Could you check a few things on this model? Use its own coordinates, in mm. A direction names the side the tool comes from. Coordinates: 2 decimals unless noted, no trailing zeros. Write each loop counter-clockwise with the first axis right and the second up, starting at its lowest first coordinate (ties: lowest second). Pieces come first, ordered by that corner, then holes.
Item 1: Thinking about a two-plate mould opening in Y: for faces 4 (the flat face through (-38.1, 65.4, 39.9)), 5 (the cylindrical face through (-31.839, -60.47, -46.367)), which applies, +Y half, -Y half, draft (parallel to the pull), parting line (faces both ways), or undercut?
Item 2: For P1, Ø12, axis at y = 63.5, z = -82.5, coming from the +X side; P2, Ø1.5, axis at x = -15.5, y = 2, coming from the -Z side; P3, Ø2, axis at x = 11.5, y = -23, coming from the -Z side; P4, Ø9.5, axis at y = 0, z = 0, coming from the -X side, each with a flat end and sliding along its axis, tell me the tip position at first contact or that it passes through.
Item 3: If I drill on probe 1 along X at (y, z) = (-67, 24.5); probe 2 along Z at (x, y) = (31.5, 0); probe 3 along X at (y, z) = (60, -67), over which ranges is the centre line in solid material (lowest first)?
Item 4: I want a section at C-C on x = -13.5. Please give me the cut outline in (y, z) (1 decimal), then the cut area to 3 significant figures.
Item 5: Which directions (+Z, -Z, +X, -X, +Y, -Y) give clear straight access to the entire face, cutting with the end or side of a thin tool? Please do faces 1 (the cylindrical face through (31.661, -60.47, -46.367)), 2 (the flat face through (-25.4, 16, 1)), 3 (the flat face through (38.1, 65.4, 39.9)).
from build123d import *

# Parameters (mm, degrees)
F0_R     = 127
F0_R_2   = 76.2
F1_DEPTH = 38.1
F2_R     = 38.09999
F0_R_3   = 7.9375
F3_DEPTH = 25.4


# Not quite as in the source:
# - a fillet or chamfer is up to 0.001 mm smaller than in the source, because OpenCascade refuses the exact size


with BuildPart() as f1:
    # F0 (on Right) → F1 (new body, symmetric)
    with BuildSketch(Plane.YZ):
        Circle(F0_R)
        Circle(F0_R_2, mode=Mode.SUBTRACT)
    extrude(amount=F1_DEPTH, both=True)

    # F2 (radius 38.1 in the source; OpenCascade refuses exactly that, so slightly less here)
    f2_edges = [f1.edges().sort_by_distance(p)[0] for p in [
        (38.1, -127, 0),
        (-38.1, -127, 0),
    ]]
    fillet(f2_edges, radius=F2_R)

    # F0 (on Right) → F3 (join, symmetric)
    with BuildSketch(Plane.YZ):
        Circle(F0_R_2)
        Circle(F0_R_3, mode=Mode.SUBTRACT)
    extrude(amount=F3_DEPTH, both=True)


solid = f1.part
Response values:
1. face 4: draft
1. face 5: undercut
2. P1: stops at x = 36.97
2. P2: stops at z = -124.01
2. P3: stops at z = -123.45
2. P4: passes through
3. probe 1: x = -25.4 to 25.4
3. probe 2: z = -110.33 to -76.2, 76.2 to 110.33
3. probe 3: x = -38.09 to 38.09
4. outline: circle Ø249.1 at (0, 0); hole circle Ø15.9 at (0, 0)
4. area: 48,500 mm2
5. face 1: +X
5. face 2: -X
5. face 3: +Z, -Z, +X, +Y, -Y
